Design review of the part built by this model. Coordinates are the model's own, in mm. Face numbers are marked on the shaded views. A direction names the side the tool comes from. Coordinates: 2 decimals unless noted, no trailing zeros. Loops run counter-clockwise (first coordinate to the right, second up) from the corner with the lowest first, then second, coordinate; pieces in that order, holes last. Notation, with made-up numbers: (56.25, -10) -> (96.25, -10) arc R15 cw to (96.25, 11) -> close; hole circle Ø6 at (30.25, 31.25). An arc over 180 degrees is marked (long way). One line per item, written item: value. Start each with the question number.
1. Machinability: for the marked faces 1, 2 and 3, which of the approach directions +Z, -Z, +X, -X, +Y, -Y give a long, thin tool a straight path to every point of the face, cutting with its end or side? Answer none if there is none.
2. For probe 1 along X at (y, z) = (-25, 26.5); probe 2 along X at (y, z) = (-5, 41); probe 3 along Y at (x, z) = (-12, 6.5), list the stretches that pass through material, from the lowest coordinate up.
3. Draft analysis for pull direction Y (two halves, no side actions). For the marked faces 4, 5, 6 and 7, state which applies: pulls with the +Y half, pulls with the -Y half, needs draft (parallel to the pull), parting line crosses it, or undercut.
4. Insertion check: pin 1 (15 mm diameter, centred on y = 4, z = 45.5, fed in from +X); pin 2 (1.5 mm diameter, centred on y = 12.5, z = 48.5, fed in from -X); pin 3 (4 mm diameter, centred on x = 3.5, y = -7.5, fed in from -Z); pin 4 (1 mm diameter, centred on x = -23.5, y = 10, fed in from +Z). Each pin has a flat end and moves straight along its axis. Give the tip position at first contact, or say it passes through.
5. Add section B-B on x = -40. Write out the cut boundary in (y, z).
6. Add section C-C on y = -5. Write out the cut boundary in (x, z), plus the area to 3 significant figures.
7. Add section D-D on x = -5.5. Write out the cut boundary in (y, z).
8. Add section A-A on z = 32.5. Write out the cut boundary in (x, y).
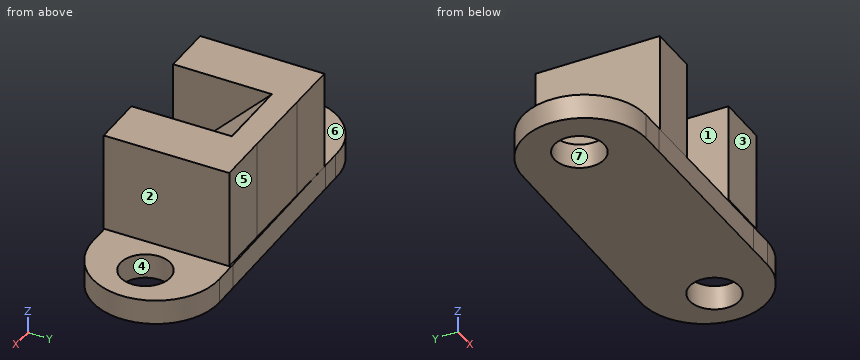
```python
from build123d import *

# Parameters (mm, degrees)
F1_DEPTH  = 12.7
F2_W      = 25.6720799953
F2_H      = 50.7660422802
F3_DEPTH  = 63.5
F5_DEPTH  = 50.7660422802
F6_W      = 26.5199552193
F6_H      = 64.0474567351
F7_DEPTH  = 50.8
F10_R     = 12.7730811137
F11_DEPTH = 63.4670422802
F12_R     = 12.7195807683
F13_DEPTH = 12.701


with BuildPart() as f1:
    # F0 (on Top) → F1 (new body)
    with BuildSketch(Plane.XY):
        with BuildLine():
            ThreePointArc((-25.6409262814, 31.6378357737), (-58.9331206672, 1.2217878444), (-28.0842930079, -31.6697917879))
            Line((-28.0842930079, -31.6697917879), (-15.4401324445, -31.7423005202))
            Line((-15.4401324445, -31.7423005202), (-15.8297911107, 31.6980969637))
            Line((-15.8297911107, 31.6980969637), (-25.6409262814, 31.6378357737))
        make_face()
        with BuildLine():
            Line((87.1467143297, 32.3305912316), (73.7005600104, 32.2480033102))
            Line((73.7005600104, 32.2480033102), (74.0967499711, -32.2557553919))
            Line((74.0967499711, -32.2557553919), (87.1467143297, -32.3305912316))
            ThreePointArc((87.1467143297, -32.3305912316), (119.4773055613, 0), (87.1467143297, 32.3305912316))
        make_face()
        Polygon((-15.8297911107, 31.6980969637), (-15.4401324445, -31.7423005202), (10.3389963129, -31.890132552), (74.0967499711, -32.2557553919), (73.7005600104, 32.2480033102), align=None)
    extrude(amount=F1_DEPTH)

    # F2 (on face) → F3 (join)
    with BuildSketch(Plane(origin=(-0.182529964, -31.8297961992, 0), x_dir=(0.9999835578, -0.0057344685, 0), z_dir=(-0.0057344685, -0.9999835578, 0))):
        with Locations((-1.8538236618, 38.0830211401)):
            Rectangle(F2_W, F2_H)
    extrude(amount=-F3_DEPTH)

    # F4 (on face) → F5 (join, through all)
    with BuildSketch(Plane.XY.offset(63.4660422802)):
        Polygon((49.3144159303, 31.3874045549), (11.1636445481, 31.6061825478), (11.0895372501, 18.6832621694), (49.3144159303, 18.6832621694), align=None)
    extrude(amount=-F5_DEPTH)

    # F6 (on face) → F7 (join)
    with BuildSketch(Plane.XY.offset(63.4660422802)):
        with Locations((62.5743935399, -0.6363238127)):
            Rectangle(F6_W, F6_H)
    extrude(amount=-F7_DEPTH)

    # F8 (on face) → F9 (join, up to the next surface of F1)
    with BuildSketch(Plane(origin=(10.982035764, -0.0629771733, 0), x_dir=(0.0057344685, 0.9999835578, 0), z_dir=(0.9999835578, -0.0057344685, 0))):
        Polygon((18.7465475772, 12.6999999999), (18.7465475772, 63.4660422802), (-31.8303195597, 12.7), align=None)
    extrude(until=Until.NEXT)

    # F10 (on face) → F11 (cut, through all)
    with BuildSketch(Plane.XY.offset(63.4660422802)):
        with Locations((-32.2718322277, 0)):
            Circle(F10_R)
    extrude(amount=-F11_DEPTH, mode=Mode.SUBTRACT)

    # F12 (on face) → F13 (cut, through all)
    with BuildSketch(Plane.XY.offset(12.7)):
        with Locations((96.3716953993, -0.4391576674)):
            Circle(F12_R)
    extrude(amount=-F13_DEPTH, mode=Mode.SUBTRACT)


solid = f1.part
```
Worked answers:
1. face 1: +Z, -Y
1. face 2: +Z, +X, +Y, -Y
1. face 3: +Z, -Z, +X, -X, -Y
2. probe 1: x = -14.83 to 10.84, 49.31 to 75.83
2. probe 2: x = -14.72 to 10.95, 49.31 to 75.83
2. probe 3: y = -31.76 to 31.72
3. face 4: undercut
3. face 5: pulls with the +Y half
3. face 6: needs draft
3. face 7: undercut
4. pin 1: stops at x = 75.83
4. pin 2: stops at x = -14.62
4. pin 3: stops at z = 0
4. pin 4: stops at z = 12.7
5. outline: (-29.01, 0) -> (-10.17, 0) -> (-10.17, 12.7) -> (-29.01, 12.7) -> close; (10.17, 0) -> (29.01, 0) -> (29.01, 12.7) -> (10.17, 12.7) -> close
6. outline: (-58.56, 0) -> (-44.03, 0) -> (-44.03, 12.7) -> (-58.56, 12.7) -> close; (-20.52, 0) -> (84.5, 0) -> (84.5, 12.7) -> (75.83, 12.7) -> (75.83, 63.47) -> (49.31, 63.47) -> (49.31, 39.91) -> (10.95, 39.69) -> (10.95, 63.47) -> (-14.72, 63.47) -> (-14.72, 12.7) -> (-20.52, 12.7) -> close; (108.25, 0) -> (119.09, 0) -> (119.09, 12.7) -> (108.25, 12.7) -> close
6. area: 5,350 mm²
7. outline: (-31.8, 0) -> (31.76, 0) -> (31.76, 12.7) -> (31.7, 12.7) -> (31.7, 63.47) -> (-31.8, 63.47) -> close
8. outline: (-14.87, -31.75) -> (10.8, -31.89) -> (10.91, -12.17) -> (49.31, -12.39) -> (49.31, -32.66) -> (75.83, -32.66) -> (75.83, 31.39) -> (49.31, 31.39) -> (-14.51, 31.75) -> close; hole (11.09, 18.68) -> (49.31, 18.46) -> (49.31, 18.68) -> close
